```python
from build123d import *

# Parameters (mm, degrees)
SKETCH1_R           = 14.478
BOSS_EXTRUDE1_DEPTH = 5.334
SKETCH2_R           = 1.905
CUT_EXTRUDE2_DEPTH  = 5.334
BOSS_EXTRUDE3_DEPTH = 5.334
SKETCH4_R           = 1.5
CUT_EXTRUDE4_DEPTH  = 22.158367706


with BuildPart() as part:
    # Sketch1 → Boss-Extrude1 (new body)
    with BuildSketch(Plane.XY):
        Circle(SKETCH1_R)
    extrude(amount=BOSS_EXTRUDE1_DEPTH)

    # Sketch2 → Cut-Extrude2 (cut)
    with BuildSketch(Plane.XY.offset(5.334)):
        Circle(SKETCH2_R)
    extrude(amount=-CUT_EXTRUDE2_DEPTH, mode=Mode.SUBTRACT)

    # Sketch3 → Boss-Extrude3 (add)
    with BuildSketch(Plane.XY.offset(5.334)):
        with BuildLine():
            Line((-1.295150956, 1.397), (1.295150956, 1.397))
            ThreePointArc((1.295150956, 1.397), (0, 1.905), (-1.295150956, 1.397))
        make_face()
    extrude(amount=-BOSS_EXTRUDE3_DEPTH)

    # Sketch4 → Cut-Extrude4 (cut, through all)
    with BuildSketch(Plane(origin=(0, 0, 0), x_dir=(-1, 0, 0), z_dir=(0, 0, -1))):
        with Locations((0, -7.5)):
            Circle(SKETCH4_R)
        with Locations(Location((7.5, 0, 0), (0, 0, 180))):
            Circle(SKETCH4_R)
        with Locations(Location((-7.5, 0, 0), (0, 0, 180))):
            Circle(SKETCH4_R)
        with Locations((0, 7.5)):
            Circle(SKETCH4_R)
    extrude(amount=-CUT_EXTRUDE4_DEPTH, mode=Mode.SUBTRACT)


solid = part.part
```
Geometry: final body of the model. Coordinates: model frame, mm. A direction names the side the tool comes from. Coordinates: 2 decimals unless noted, no trailing zeros. Write each loop counter-clockwise with the first axis right and the second up, starting at its lowest first coordinate (ties: lowest second). Pieces come first, ordered by that corner, then holes. Notation, with made-up numbers: M -36,40.25 L -20,40.25 A22 ccw -20,55.25 Z; hole C 37,10.5 d5. An arc over 180 degrees is marked long. Use CSV: the item, a comma, the result in double quotes. Start each with the question number.
1. Reachability of faces 1 (the face through (0, 1.397, 3)), 2 (the face through (0, -3, 5.334)) from +Z, -Z, +X, -X, +Y, -Y: full face, straight path, thin tool, end or side. Return the list, or none.
2. Ray query, probe 1 along Y at (x, z) = (0, 2.65) (3 decimals); probe 2 along X at (y, z) = (-0.5, 0.55); probe 3 along Y at (x, z) = (-7.5, 2.75). Return the intervals inside material, ascending.
3. First-contact query: P1, Ø2, axis at x = 1.5, y = 9, coming from the -Z side; P2, Ø3, axis at x = 2.5, z = 4.5, coming from the -Y side; P3, Ø2.5, axis at x = -7.5, y = 0, coming from the -Z side. Flat tips, straight axial feed; report the tip coordinate or a pass-through.
4. Cut plane B-B on z = 1.7. Return the cut outline in (x, y) (3 decimals), plus the area to 3 significant figures.
5. Cut plane A-A on x = 0. Return the cut outline in (y, z) (3 decimals), plus the area to 3 significant figures.
6. Cut plane C-C on x = 7.5. Return the cut outline in (y, z).
7. Mould query, pull axis Y, two halves, no side actions, for faces 3 (the face through (-9, 0, 3)), 4 (the face through (-1.885, 14.355, 2.63)), 5 (the face through (0, -3, 0)). Classes: pulls with the +Y half, pulls with the -Y half, needs draft (parallel to the pull), parting line crosses it, or undercut.
Entries:
1,face 1,"+Z, -Z"
1,face 2,"+Z, +X, -X, +Y, -Y"
2,probe 1,"-14.478 to -9, -6 to -1.905, 1.397 to 6, 9 to 14.478"
2,probe 2,"-14.47 to -8.91, -6.09 to -1.84, 1.84 to 6.09, 8.91 to 14.47"
2,probe 3,"-12.38 to -1.5, 1.5 to 12.38"
3,P1,"z = 0"
3,P2,"y = -14.44"
3,P3,"through"
4,outline,"C 0,0 d28.956; hole C -7.5,0 d3; hole C 0,-7.5 d3; hole C 0,7.5 d3; hole M -1.295,1.397 A1.905 ccw long 1.295,1.397 Z; hole C 7.5,0 d3"
4,area,"620 mm²"
5,outline,"M -14.478,0 L -9,0 L -9,5.334 L -14.478,5.334 Z; M -6,0 L -1.905,0 L -1.905,5.334 L -6,5.334 Z; M 1.397,0 L 6,0 L 6,5.334 L 1.397,5.334 Z; M 9,0 L 14.478,0 L 14.478,5.334 L 9,5.334 Z"
5,area,"105 mm²"
6,outline,"M -12.38,0 L -1.5,0 L -1.5,5.33 L -12.38,5.33 Z; M 1.5,0 L 12.38,0 L 12.38,5.33 L 1.5,5.33 Z"
7,face 3,"undercut"
7,face 4,"parting line crosses it"
7,face 5,"needs draft"
